Geometry: final body of the model. Coordinates: model frame, mm. A direction names the side the tool comes from. Round coordinates to 2 decimals unless told otherwise and drop trailing zeros. Write each loop counter-clockwise with the first axis right and the second up, starting at its lowest first coordinate (ties: lowest second). Pieces come first, ordered by that corner, then holes. Notation, with made-up numbers: M 88,-8.5 L 106,-8.5 A28 cw 106,19.5 Z; hole C 76.5,48 d4. An arc over 180 degrees is marked long. Answer as CSV lines item,"result". Start each with the question number.
Q1. Section query A-A on y = 40.5. Output: boundary loops of the cut face in (x, z), and give its area (3 significant figures).
Q2. Section query C-C on x = 11. Output: boundary loops of the cut face in (y, z), and give its area (3 significant figures).
Q3. Reachability of faces 4 (the flat face through (36.87, 39.55, 8.18)), 5 (the flat face through (11, 59.76, 8)) from +Z, -Z, +X, -X, +Y, -Y: full face, straight path, thin tool, end or side. Return the list, or none.
Q4. First-contact query: pin 1 (5 mm diameter, centred on y = 19, z = 6.5, fed in from +X); pin 2 (8 mm diameter, centred on x = 28.5, z = 3.5, fed in from +Y); pin 3 (3 mm diameter, centred on x = 28, z = 7, fed in from +Y). Flat tips, straight axial feed; report the tip coordinate or a pass-through.
Q5. Mould query, pull axis X, two halves, no side actions, for faces 1 (the flat face through (25.32, 53.95, 8.18)), 2 (the flat face through (-2.215, 29, 8)), 3 (the flat face through (30.187, 53.549, 8.184)). Classes: pulls with the +X half, pulls with the -X half, needs draft (parallel to the pull), parting line crosses it, or undercut.
Q6. Ray query, probe 1 along Y at (x, z) = (4.5, 10.75); probe 2 along Y at (x, z) = (27, 10.5); probe 3 along X at (y, z) = (18, 6.5). Return the intervals inside material, ascending.
Q7. Section query B-B on z = 13.75. Output: boundary loops of the cut face in (x, y), and give its area (3 significant figures).
Q8. Section query D-D on x = 41. Output: boundary loops of the cut face in (y, z).
```python
from build123d import *

# Parameters (mm, degrees)
PAD_DEPTH = 16.6


with BuildPart() as part:
    # Sketch → Pad (new body)
    with BuildSketch(Plane.XY):
        Polygon((-2.215162, 59.759811), (-2.215162, -3.075415), (38.48941, -3.075415), (45.010048, 28.539799), (36.908657, 47.508923), (23.274607, 59.759811), align=None)
        Polygon((0, 0), (35, 0), (37, 7.2), (38.5, 14.4), (39.6, 21.6), (39.7, 28.8), (38.4, 36), (35.3, 43.2), (30.5, 50.4), (20, 57.6), (0, 57.6), align=None, mode=Mode.SUBTRACT)
    extrude(amount=PAD_DEPTH)


solid = part.part
```
Entries:
1,outline,"M -2.22,0 L 0,0 L 0,16.6 L -2.22,16.6 Z; M 36.46,0 L 39.9,0 L 39.9,16.6 L 36.46,16.6 Z"
1,area,"93.9 mm^2"
2,outline,"M -3.08,0 L 0,0 L 0,16.6 L -3.08,16.6 Z; M 57.6,0 L 59.76,0 L 59.76,16.6 L 57.6,16.6 Z"
2,area,"86.9 mm^2"
3,face 4,"+Z, -Z"
3,face 5,"+Z, -Z, +X, -X, +Y"
4,pin 1,"stops at x = 43.56"
4,pin 2,"stops at y = 58.66"
4,pin 3,"stops at y = 56.86"
5,face 1,"undercut"
5,face 2,"pulls with the -X half"
5,face 3,"pulls with the +X half"
6,probe 1,"y = -3.08 to 0, 57.6 to 59.76"
6,probe 2,"y = -3.08 to 0, 52.8 to 56.41"
6,probe 3,"x = -2.22 to 0, 39.05 to 42.84"
7,outline,"M -2.22,-3.08 L 38.49,-3.08 L 45.01,28.54 L 36.91,47.51 L 23.27,59.76 L -2.22,59.76 Z; hole M 0,0 L 35,0 L 37,7.2 L 38.5,14.4 L 39.6,21.6 L 39.7,28.8 L 38.4,36 L 35.3,43.2 L 30.5,50.4 L 20,57.6 L 0,57.6 Z"
7,area,"542 mm^2"
8,outline,"M 9.1,0 L 37.93,0 L 37.93,16.6 L 9.1,16.6 Z"
